from build123d import *

# Parameters (mm, degrees)
F0_W     = 96.598558
F0_H     = 94.948866
F1_DEPTH = 38.1
F2_R     = 24.762498
F3_DEPTH = 33.274
F5_DEPTH = 635


with BuildPart() as f1:
    # F0 (on Front) → F1 (new body)
    with BuildSketch(Plane.XZ):
        Rectangle(F0_W, F0_H)
    extrude(amount=F1_DEPTH)

    # F2 (on face) → F3 (join)
    with BuildSketch(Plane.XZ.offset(38.1)):
        Circle(F2_R)
    extrude(amount=F3_DEPTH)

    # F4 (on Right) → F5 (cut, symmetric)
    with BuildSketch(Plane.YZ):
        Polygon((-71.105659, 24.648242), (-71.105659, -24.648242), (-38.585469, 24.648242), align=None)
    extrude(amount=F5_DEPTH, both=True, mode=Mode.SUBTRACT)


solid = f1.part
Can you work these out from the model? Positions are in its coordinate system, mm. A direction names the side the tool comes from. Coordinates: 2 decimals unless noted, no trailing zeros. Write each loop counter-clockwise with the first axis right and the second up, starting at its lowest first coordinate (ties: lowest second). Pieces come first, ordered by that corner, then holes. Notation, with made-up numbers: (12, -18) - (57, -18) arc R12 cw to (57, -13) - close; hole circle Ø5 at (-38, 25). An arc over 180 degrees is marked (long way). Return JSON: item names as keys, results as strings. Group by question number.
Item 1: If we section it at B-B (z = -15): Write out the boundary of the cut face in (x, y).
Item 2: If we section it at A-A (x = 0): Write out the boundary of the cut face in (y, z), then the cut area to 3 significant figures.
Item 3: Which directions (+Z, -Z, +X, -X, +Y, -Y) give clear straight access to the entire face, cutting with the end or side of a thin tool? Please do faces 4 (the face through (48.299, -19, -1)), 5 (the face through (-22, -38.1, 22)).
Item 4: I'm going to push flat-ended pins straight in: pin 1 Ø4 at (x, z) = (37.5, -11) entering from -Y; pin 2 Ø4 at (x, z) = (-10.5, 9.5) entering from +Y; pin 3 Ø2.5 at (x, y) = (0.5, -54.5) entering from -Z. Where does each tip first touch, or does it pass through?
Item 5: We'd pull the mould along Y, two halves only. Please class faces 1 (the face through (-1, 0, 1)), 2 (the face through (0, -71.374, 0)), 3 (the face through (0.347, -55.073, -0.345)): pulls with the +Y half, pulls with the -Y half, needs draft (parallel to the pull), parting line crosses it, or undercut.
Item 6: If we section it at D-D (y = -50): Write out the boundary of the cut face in (x, z) (1 decimal), then the cut area to 3 significant figures.
Item 7: Please list where these lines run through material, in increasing order: probe 1 along Y at (x, z) = (10, -24.5); probe 2 along X at (y, z) = (-49, -18); probe 3 along Z at (x, y) = (-4.5, -65.5).
Item 8: If we section it at C-C (x = 11): Write out the boundary of the cut face in (y, z).
Return value:
{
 "1": {"outline": "(-48.3, -38.1) - (-19.7, -38.1) - (-19.7, -64.74) - (19.7, -64.74) - (19.7, -38.1) - (48.3, -38.1) - (48.3, 0) - (-48.3, 0) - close; (-19.7, -71.37) - (19.7, -71.37) - (19.7, -71.11) - (-19.7, -71.11) - close"},
 "2": {"outline": "(-71.37, -24.76) - (-38.1, -24.76) - (-38.1, -47.47) - (0, -47.47) - (0, 47.47) - (-38.1, 47.47) - (-38.1, 24.76) - (-71.37, 24.76) - close; hole (-71.11, -24.65) - (-38.59, 24.65) - (-71.11, 24.65) - close", "area": "4,460 mm^2"},
 "3": {"face 4": "+Z, -Z, +X, +Y, -Y", "face 5": "-Y"},
 "4": {"pin 1": "stops at y = -38.1", "pin 2": "stops at y = 0", "pin 3": "stops at z = -24.76"},
 "5": {"face 1": "pulls with the +Y half", "face 2": "pulls with the -Y half", "face 3": "undercut"},
 "6": {"outline": "(-23.6, 7.3) arc R24.8 ccw (long way) to (23.6, 7.3) - close; (-2.4, 24.6) - (2.4, 24.6) arc R24.8 ccw to start", "area": "1,320 mm^2"},
 "7": {"probe 1": "y = -38.1 to 0", "probe 2": "x = -17.01 to 17.01", "probe 3": "z = -24.35 to -16.15"},
 "8": {"outline": "(-71.37, -22.19) - (-71.11, -22.19) - (-71.11, 22.19) - (-71.37, 22.19) - close; (-69.48, -22.19) - (-38.1, -22.19) - (-38.1, -47.47) - (0, -47.47) - (0, 47.47) - (-38.1, 47.47) - (-38.1, 22.19) - (-40.21, 22.19) - close"}
}
